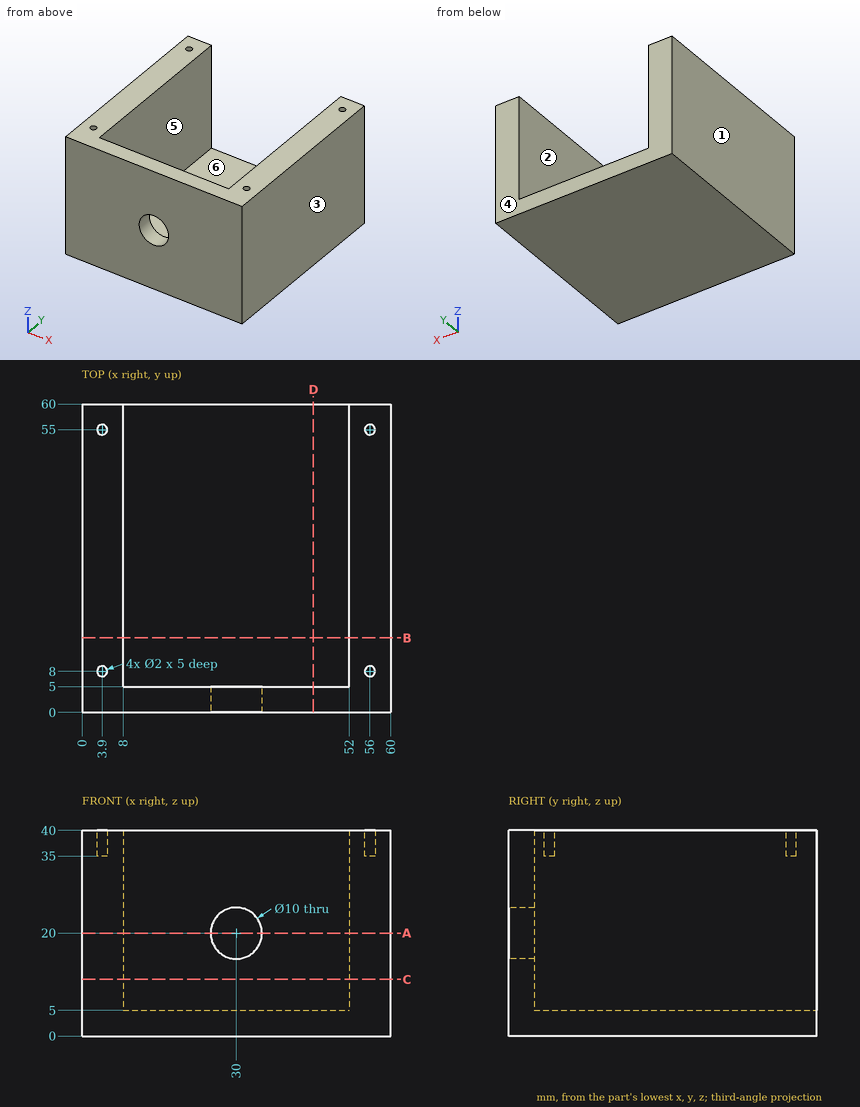
The figure shows three views and two pictorial views of one solid part (mm, origin at its lowest corner). Answer the questions. A direction names the side the tool comes from. Round coordinates to 2 decimals unless told otherwise and drop trailing zeros. Order: outer loops, then holes, each group sorted by start corner. A loop starts at its lowest first (then second) coordinate and runs counter-clockwise, first axis right, second up. Notation, with made-up numbers: M 36,14.25 L 55,14.25 A34 ccw 55,51.25 Z; hole C 21,71 d8. An arc over 180 degrees is marked long. Put each result on its own line as item: value. Start each with the question number.
Q1. Straight lines are drawn through the part: L1, parallel to Y at x = 56, z = 36; L2, parallel to X at y = 41, z = 22.5; L3, parallel to Z at x = 46.5, y = 26.5. For each, find the intervals that lie inside material, in ascending order. Write a range as [from, to].
Q2. Section C-C, the plane z = 11 is taken. Write down the section's boundary in (x, y).
Q3. Section D-D, the plane x = 45 is taken. Write down the section's boundary in (y, z).
Q4. A tool of negligible diameter and unlimited length cuts with its end or side. For the marked faces 1 and 2, from which of +Z, -Z, +X, -X, +Y, -Y can it reach the whole face along a straight path? Write none if from no direction.
Q5. For a pull along X with two mould halves and no side action, classify the marked faces 3, 4, 5 and 6 as pulls with the +X half, pulls with the -X half, needs draft (parallel to the pull), parting line crosses it, or undercut.
Q6. Section B-B, the plane y = 14.5 is taken. Write down the section's boundary in (x, z), and give its area (3 significant figures).
Q7. Section A-A, the plane z = 20 is taken. Write down the section's boundary in (x, y).
Q8. Flat-ended cylindrical pins translate along their axes: pin 1 (1.8 mm diameter, centred on x = 56, y = 8, fed in from +Z); pin 2 (2 mm diameter, centred on x = 46, z = 36, fed in from +Y). Find the tip coordinate at first contact, or state that the pin passes through.
Findings below:
1. L1: y = [0, 7], [9, 54], [56, 60]
1. L2: x = [0, 8], [52, 60]
1. L3: z = [0, 5]
2. outline: M 0,0 L 60,0 L 60,60 L 52,60 L 52,5 L 8,5 L 8,60 L 0,60 Z
3. outline: M 0,0 L 60,0 L 60,5 L 5,5 L 5,40 L 0,40 Z
4. face 1: +Z, -Z, -X, +Y, -Y
4. face 2: +Z, +Y
5. face 3: pulls with the +X half
5. face 4: needs draft
5. face 5: undercut
5. face 6: undercut
6. outline: M 0,0 L 60,0 L 60,40 L 52,40 L 52,5 L 8,5 L 8,40 L 0,40 Z
6. area: 860 mm^2
7. outline: M 0,0 L 25,0 L 25,5 L 8,5 L 8,60 L 0,60 Z; M 35,0 L 60,0 L 60,60 L 52,60 L 52,5 L 35,5 Z
8. pin 1: stops at z = 35
8. pin 2: stops at y = 5
